from build123d import *

# Parameters (mm, degrees)
SKETCH_1_R          = 14
EXTRUDE_1_DEPTH     = 19
SKETCH_3_R          = 4
EXTRUDE_2_DEPTH     = 1.8
SKETCH_4_R          = 2.5
EXTRUDE_3_DEPTH     = 8.2
SKETCH_5_R          = 2
EXTRUDE_4_DEPTH     = 1
CUT_EXTRUDE_START   = -8.2
CUT_EXTRUDE_1_DEPTH = 8.2


with BuildPart() as part:
    # 草图1 → 凸台-拉伸1 (new body)
    with BuildSketch(Plane.XY):
        Circle(SKETCH_1_R)
    extrude(amount=EXTRUDE_1_DEPTH)

    # 草图3 → 凸台-拉伸2 (add)
    with BuildSketch(Plane.XY):
        with Locations((0, 6.835245796)):
            Circle(SKETCH_3_R)
    extrude(amount=-EXTRUDE_2_DEPTH)

    # 草图4 → 凸台-拉伸3 (add)
    with BuildSketch(Plane(origin=(0, 0, -1.8), x_dir=(-1, 0, 0), z_dir=(0, 0, -1))):
        with Locations((0, 6.835245796)):
            Circle(SKETCH_4_R)
    extrude(amount=EXTRUDE_3_DEPTH)

    # 草图5 → 凸台-拉伸4 (add)
    with BuildSketch(Plane(origin=(0, 0, 0), x_dir=(-1, 0, 0), z_dir=(0, 0, -1))):
        with BuildLine():
            Line((-17.5, 4), (17.5, 4))
            ThreePointArc((17.5, 4), (21.5, 0), (17.5, -4))
            Line((17.5, -4), (-17.5, -4))
            ThreePointArc((-17.5, -4), (-21.5, 0), (-17.5, 4))
        make_face()
        with Locations((17.5, 0)):
            Circle(SKETCH_5_R, mode=Mode.SUBTRACT)
        with Locations((-17.5, 0)):
            Circle(SKETCH_5_R, mode=Mode.SUBTRACT)
    extrude(amount=-EXTRUDE_4_DEPTH)

    # 草图6 → 切除-拉伸1 (cut)
    with BuildSketch(Plane(origin=(0, 0, -10), x_dir=(-1, 0, 0), z_dir=(0, 0, -1)).offset(CUT_EXTRUDE_START)):
        with BuildLine():
            Line((-1.5, 8.835245796), (1.5, 8.835245796))
            ThreePointArc((1.5, 8.835245796), (0, 9.335245796), (-1.5, 8.835245796))
        make_face()
        with BuildLine():
            Line((1.5, 4.835245796), (-1.5, 4.835245796))
            ThreePointArc((-1.5, 4.835245796), (0, 4.335245796), (1.5, 4.835245796))
        make_face()
    extrude(amount=CUT_EXTRUDE_1_DEPTH, mode=Mode.SUBTRACT)


solid = part.part
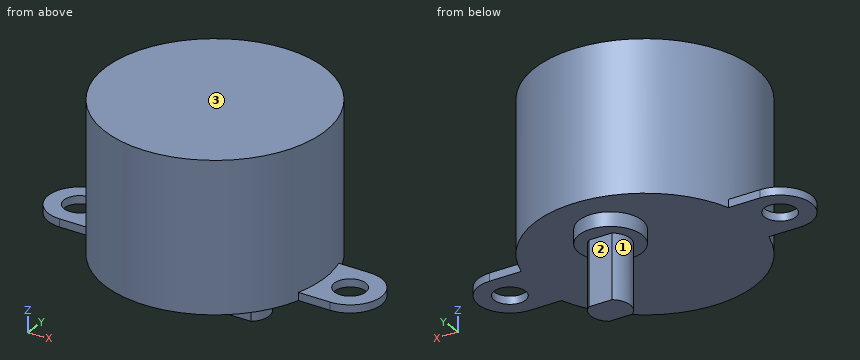
Source: CAD feature listing. Evaluate the final solid. Frame: model axes, mm. Face numbers are marked on the shaded views. A direction names the side the tool comes from. Coordinates: 2 decimals unless noted, no trailing zeros. Loops run counter-clockwise (first coordinate to the right, second up) from the corner with the lowest first, then second, coordinate; pieces in that order, holes last. Notation, with made-up numbers: (-31, 86.5) -> (25, 86.5) arc R11 ccw to (25, 95.5) -> close; hole circle Ø11 at (-6, 85.5). An arc over 180 degrees is marked (long way). Answer in a Markdown table with one row per item. Add a question column.
Q1. Section B-B on x = -2. Return the cut outline in (y, z).
Q2. Reachability of the marked faces 1, 2 and 3 from +Z, -Z, +X, -X, +Y, -Y: full face, straight path, thin tool, end or side. Return the list, or none.
Q3. Section D-D on y = 8.25. Return the cut outline in (x, z), and give its area (3 significant figures).
Q4. Contact query for flat-ended pins moving along their axis: pin 1 Ø2.5 at (x, z) = (-0.5, -8) entering from -Y; pin 2 Ø2 at (x, y) = (-4.5, 11) entering from -Z; pin 3 Ø10 at (y, z) = (-6.5, 9.5) entering from -X. Output: stop coordinate, or through.
Q5. Section A-A on y = 0. Return the cut outline in (x, z).
Q6. Ray query, line 1 along Y through (x, z) = (-17.5, 0.5); line 2 along Z through (x, y) = (-6.5, 11.25); line 3 along Z through (x, y) = (16, 1.75). Return the intervals inside material, ascending.
Q7. Section C-C on z = 4. Return the cut outline in (x, y).
Computed values:
| question | item | result |
|---|---|---|
| 1 | outline | (-13.86, 0) -> (3.37, 0) -> (3.37, -1.8) -> (5.34, -1.8) -> (5.34, -10) -> (8.34, -10) -> (8.34, -1.8) -> (10.3, -1.8) -> (10.3, 0) -> (13.86, 0) -> (13.86, 19) -> (-13.86, 19) -> close |
| 2 | face 1 | -Z, -X |
| 2 | face 2 | -Z, +X, -X, +Y |
| 2 | face 3 | +Z, +X, -X, +Y, -Y |
| 3 | outline | (-11.31, 0) -> (-3.74, 0) -> (-3.74, -1.8) -> (-2.06, -1.8) -> (-2.06, -10) -> (2.06, -10) -> (2.06, -1.8) -> (3.74, -1.8) -> (3.74, 0) -> (11.31, 0) -> (11.31, 19) -> (-11.31, 19) -> close |
| 3 | area | 477 mm^2 |
| 4 | pin 1 | stops at y = 4.84 |
| 4 | pin 2 | stops at z = 0 |
| 4 | pin 3 | stops at x = -13.92 |
| 5 | outline | (-21.5, 0) -> (-19.5, 0) -> (-19.5, 1) -> (-21.5, 1) -> close; (-15.5, 0) -> (15.5, 0) -> (15.5, 1) -> (14, 1) -> (14, 19) -> (-14, 19) -> (-14, 1) -> (-15.5, 1) -> close; (19.5, 0) -> (21.5, 0) -> (21.5, 1) -> (19.5, 1) -> close |
| 6 | line 1 | y = -4 to -2, 2 to 4 |
| 6 | line 2 | z = 0 to 19 |
| 6 | line 3 | z = 0 to 1 |
| 7 | outline | circle Ø28 at (0, 0) |
